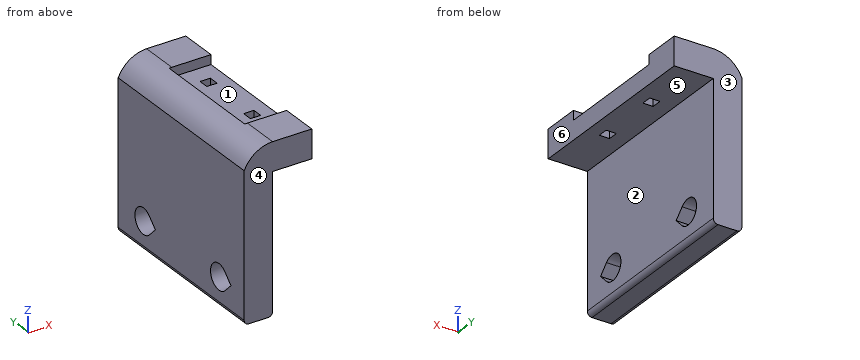
from build123d import *

# Parameters (mm, degrees)
BOSS_EXTRUDE1_DEPTH = 100
CUT_EXTRUDE1_DEPTH  = 126.693414536
SKETCH3_W           = 5.4
SKETCH3_H           = 5.4
CUT_EXTRUDE2_DEPTH  = 139.050096295
SKETCH4_W           = 22
SKETCH4_H           = 60
CUT_EXTRUDE3_DEPTH  = 5
FILLET1_R           = 2.5


with BuildPart() as part:
    # Sketch1 → Boss-Extrude1 (new body)
    with BuildSketch(Plane(origin=(0, 0, 0), x_dir=(-1, 0, 0), z_dir=(0, 1, 0))):
        with BuildLine():
            Line((-16.539379475, 20.305108986), (-16.462740437, 20.305108986))
            ThreePointArc((-16.462740437, 20.305108986), (-7.525387839, 17.507307751), (-1.539379475, 10.305108986))
            Line((-1.539379475, 10.305108986), (-1.539379475, -67.344891014))
            Line((-1.539379475, -67.344891014), (-16.539379475, -67.344891014))
            Line((-16.539379475, -67.344891014), (-16.539379475, 5.305108986))
            Line((-16.539379475, 5.305108986), (-37.085126223, 5.305108986))
            Line((-37.085126223, 5.305108986), (-37.085126223, 20.305108986))
            Line((-37.085126223, 20.305108986), (-16.539379475, 20.305108986))
        make_face()
    extrude(amount=BOSS_EXTRUDE1_DEPTH)

    # Sketch2 → Cut-Extrude1 (cut, through all)
    with BuildSketch(Plane(origin=(1.539379475, 0, 0), x_dir=(0, -1, 0), z_dir=(-1, 0, 0))):
        with BuildLine():
            Line((-75.262384566, -47.60727558), (-70.524769132, -52.344891014))
            Line((-70.524769132, -52.344891014), (-75.262384566, -57.082506448))
            ThreePointArc((-75.262384566, -57.082506448), (-86.7, -52.344891014), (-75.262384566, -47.60727558))
        make_face()
        with BuildLine():
            Line((-10.524769132, -52.344891014), (-15.262384566, -47.60727558))
            ThreePointArc((-15.262384566, -47.60727558), (-26.7, -52.344891014), (-15.262384566, -57.082506448))
            Line((-15.262384566, -57.082506448), (-10.524769132, -52.344891014))
        make_face()
    extrude(amount=-CUT_EXTRUDE1_DEPTH, mode=Mode.SUBTRACT)

    # Sketch3 → Cut-Extrude2 (cut, through all)
    with BuildSketch(Plane.XY.offset(20.305108986)):
        with Locations((27.385126223, 32.7)):
            Rectangle(SKETCH3_W, SKETCH3_H)
        with Locations((27.385126223, 67.3)):
            Rectangle(SKETCH3_W, SKETCH3_H)
    extrude(amount=-CUT_EXTRUDE2_DEPTH, mode=Mode.SUBTRACT)

    # Sketch4 → Cut-Extrude3 (cut)
    with BuildSketch(Plane.XY.offset(20.305108986)):
        with Locations((26.085126223, 50)):
            Rectangle(SKETCH4_W, SKETCH4_H)
    extrude(amount=-CUT_EXTRUDE3_DEPTH, mode=Mode.SUBTRACT)

    # Fillet1
    fillet1_edges = [part.edges().sort_by_distance(p)[0] for p in [
        (1.539379475, 50, -67.344891014),
        (16.539379475, 50, -67.344891014),
    ]]
    fillet(fillet1_edges, radius=FILLET1_R)


solid = part.part
CAD build for the part. Positions are in the model's coordinates, mm. Face numbers are marked on the shaded views. A direction names the side the tool comes from. Round coordinates to 2 decimals unless told otherwise and drop trailing zeros. Write each loop counter-clockwise with the first axis right and the second up, starting at its lowest first coordinate (ties: lowest second). Pieces come first, ordered by that corner, then holes.
(1) Mould opens along Y. For the marked faces 1, 2, 3 and 4 say: pulls with the +Y half, pulls with the -Y half, needs draft (parallel to the pull), parting line crosses it, or undercut.
(2) Drop flat-ended pins along their axis: P1, Ø3, axis at x = 15.5, y = 57, coming from the +Z side; P2, Ø3, axis at y = 87.5, z = -15, coming from the +X side; P3, Ø4, axis at y = 62, z = 17, coming from the +X side; P4, Ø10.5, axis at x = 30.5, y = 64.5, coming from the -Z side. Give the stop position or say it passes through.
(3) Slice it at C-C, the plane y = 52. Write the cut outline in (x, z), and give its area (3 significant figures).
(4) Probe line 1 along Y through (x, z) = (14, -57.5); line 2 along X through (y, z) = (79.5, -9.5); line 3 along Z through (x, y) = (29.5, 28.5). List the from-to ranges inside material, lowest first.
(5) Slice it at D-D, the plane z = -11. Write the cut outline in (x, y), and give its area (3 significant figures).
(6) Slice it at B-B, the plane x = 6. Write the cut outline in (y, z), and give its area (3 significant figures).
(7) 3-axis set-ups, long thin cutter, end or side, ignore diameter. For the marked faces 5 and 6: which of +Z, -Z, +X, -X, +Y, -Y reach the whole face in a straight line?
(8) Slice it at A-A, the plane y = 76.5. Write the cut outline in (x, z), and give its area (3 significant figures).
From the geometry:
1. face 1: undercut
1. face 2: needs draft
1. face 3: pulls with the +Y half
1. face 4: pulls with the -Y half
2. P1: stops at z = 20.22
2. P2: stops at x = 16.54
2. P3: stops at x = 37.09
2. P4: stops at z = 5.31
3. outline: (1.54, -64.84) arc R2.5 ccw to (4.04, -67.34) - (14.04, -67.34) arc R2.5 ccw to (16.54, -64.84) - (16.54, 5.31) - (37.09, 5.31) - (37.09, 15.31) - (15.09, 15.31) - (15.09, 20.22) arc R16.54 ccw to (1.54, 10.31) - close
3. area: 1,470 mm2
4. line 1: y = 0 to 15.72, 24.28 to 75.72, 84.28 to 100
4. line 2: x = 1.54 to 16.54
4. line 3: z = 5.31 to 15.31
5. outline: (1.54, 0) - (16.54, 0) - (16.54, 100) - (1.54, 100) - close
5. area: 1,500 mm2
6. outline: (0, -67.34) - (100, -67.34) - (100, 16.35) - (0, 16.35) - close; hole (10.52, -52.34) - (15.26, -57.08) arc R6.7 ccw (long way) to (15.26, -47.61) - close; hole (70.52, -52.34) - (75.26, -57.08) arc R6.7 ccw (long way) to (75.26, -47.61) - close
6. area: 8,070 mm2
7. face 5: -Z, +X, +Y, -Y
7. face 6: +Z, -Z, +X, +Y, -Y
8. outline: (1.54, -64.84) arc R2.5 ccw to (4.04, -67.34) - (14.04, -67.34) arc R2.5 ccw to (16.54, -64.84) - (16.54, -58.06) - (1.54, -58.06) - close; (1.54, -46.63) - (16.54, -46.63) - (16.54, 5.31) - (37.09, 5.31) - (37.09, 15.31) - (15.09, 15.31) - (15.09, 20.22) arc R16.54 ccw to (1.54, 10.31) - close
8. area: 1,300 mm2
